from build123d import *

# Parameters (mm, degrees)
F0_W     = 50.8
F0_H     = 76.2
F1_DEPTH = 50.8
F2_T     = -12.7
F3_W     = 12.7
F3_H     = 25.4
F4_DEPTH = 38.1


with BuildPart() as f1:
    # F0 (on Front) → F1 (new body)
    with BuildSketch(Plane.XZ):
        with Locations((25.4, -38.1)):
            Rectangle(F0_W, F0_H)
    extrude(amount=F1_DEPTH)

    # F2
    f2_openings = [f1.faces().sort_by_distance(p)[0] for p in [
        (25.4, -50.8, -38.1),
        (25.4, -25.4, 0),
    ]]
    offset(amount=F2_T, openings=f2_openings)

    # F3 (on face) → F4 (cut)
    with BuildSketch(Plane.XZ.offset(12.7)):
        with Locations((6.35, -12.7)):
            Rectangle(F3_W, F3_H)
        with Locations((44.45, -12.7)):
            Rectangle(F3_W, F3_H)
    extrude(amount=F4_DEPTH, mode=Mode.SUBTRACT)


solid = f1.part
Input: part model. Units: mm. Frame: model coordinates. A direction names the side the tool comes from. Give positions to 0.01 mm unless a question says otherwise; leave off trailing zeros. Order: outer loops, then holes, each group sorted by start corner. A loop starts at its lowest first (then second) coordinate and runs counter-clockwise, first axis right, second up. Notation, with made-up numbers: (87.25, 78) - (134.25, 78) arc R31 cw to (134.25, 108) - close; hole circle Ø7 at (36, -37.75). An arc over 180 degrees is marked (long way). Write each question's results on one line, items separated by ' | '.
Item 1: Contact query for flat-ended pins moving along their axis: pin 1 Ø10 at (y, z) = (-26.5, -18) entering from -X; pin 2 Ø4 at (x, y) = (5, -37) entering from +Z; pin 3 Ø6 at (x, z) = (19.5, -19.5) entering from -Y. Output: stop coordinate, or through.
A:
pin 1: passes through | pin 2: stops at z = -25.4 | pin 3: stops at y = -12.7
Item 2: Draft query along X for faces 4 (the flat face through (25, -12.7, -24)), 5 (the flat face through (50.8, -25, -47)), 6 (the flat face through (6, -31, -25.4)), 7 (the flat face through (12.7, -31, -45)). Return one class per face: released by +X, released by -X, zero draft, split by the parting line, or undercut.
A:
face 4: undercut | face 5: released by +X | face 6: zero draft | face 7: undercut
Item 3: Section A-A (y = -44.5). Return loops of the section in (x, z), and give its area (3 significant figures).
A:
outline: (0, -76.2) - (50.8, -76.2) - (50.8, -25.4) - (38.1, -25.4) - (38.1, -63.5) - (12.7, -63.5) - (12.7, -25.4) - (0, -25.4) - close | area: 1,610 mm^2
Item 4: Section B-B (x = 18.5). Return loops of the section in (y, z).
A:
outline: (-50.8, -76.2) - (0, -76.2) - (0, 0) - (-12.7, 0) - (-12.7, -63.5) - (-50.8, -63.5) - close
Item 5: Access query for faces 1 (the flat face through (25, 0, -38)), 2 (the flat face through (38.1, -31, -45)), 3 (the flat face through (44, -31, -25.4)). Directions: +Z, -Z, +X, -X, +Y, -Y. A direction counts if a zero-diameter tool reaches every point of the face in a straight line with its end or side. Return the directions, or none.
A:
face 1: +Z, -Z, +X, -X, +Y | face 2: +Z, -Y | face 3: +Z, +X, -X, -Y
Item 6: Material intervals for line 1 along X through (y, z) = (-36.5, -29.5); line 2 along Z through (x, y) = (13, -14); line 3 along Y through (x, z) = (22.5, -18), sorted ascending.
A:
line 1: x = 0 to 12.7, 38.1 to 50.8 | line 2: z = -76.2 to -63.5 | line 3: y = -12.7 to 0
Item 7: Section D-D (x = 45). Return loops of the section in (y, z).
A:
outline: (-50.8, -76.2) - (0, -76.2) - (0, 0) - (-12.7, 0) - (-12.7, -25.4) - (-50.8, -25.4) - close
Item 8: Section C-C (z = -56.5). Return loops of the section in (x, y).
A:
outline: (0, -50.8) - (12.7, -50.8) - (12.7, -12.7) - (38.1, -12.7) - (38.1, -50.8) - (50.8, -50.8) - (50.8, 0) - (0, 0) - close
